```python
from build123d import *

# Parameters (mm, degrees)
SKETCH1_W           = 40
SKETCH1_H           = 45
BOSS_EXTRUDE1_DEPTH = 50
SHELL1_T            = -2.5
SKETCH3_W           = 40
SKETCH3_H           = 34.5
BOSS_EXTRUDE2_DEPTH = 10
SKETCH11_W          = 40
SKETCH11_H          = 5
CUT_EXTRUDE2_DEPTH  = 2.5
SKETCH12_W          = 37.5
SKETCH12_H          = 2
CUT_EXTRUDE3_DEPTH  = 1
SKETCH13_W          = 37.5
SKETCH13_H          = 2
CUT_EXTRUDE4_DEPTH  = 1
SKETCH15_R          = 1.5
CUT_EXTRUDE7_DEPTH  = 37
SKETCH16_R          = 1.5
CUT_EXTRUDE8_DEPTH  = 37
SKETCH17_R          = 3
CUT_EXTRUDE9_DEPTH  = 5
SKETCH19_W          = 15
SKETCH19_H          = 15
CUT_EXTRUDE10_DEPTH = 2.5


with BuildPart() as part:
    # Sketch1 → Boss-Extrude1 (new body)
    with BuildSketch(Plane(origin=(0, 0, 0), x_dir=(1, 0, 0), z_dir=(0, 1, 0))):
        with Locations((-14.888700463, -8.449653636)):
            Rectangle(SKETCH1_W, SKETCH1_H)
    extrude(amount=BOSS_EXTRUDE1_DEPTH)

    # Shell1
    shell1_openings = [part.faces().sort_by_distance(p)[0] for p in [
        (-14.888700463, 50, 8.449653636),
    ]]
    offset(amount=SHELL1_T, openings=shell1_openings, kind=Kind.INTERSECTION)

    # Sketch3 → Boss-Extrude2 (add)
    with BuildSketch(Plane(origin=(-32.388700463, 0, 0), x_dir=(0, 0, -1), z_dir=(1, 0, 0))):
        with Locations((-8.449653636, 19.75)):
            Rectangle(SKETCH3_W, SKETCH3_H)
    extrude(amount=BOSS_EXTRUDE2_DEPTH)

    # Sketch11 → Cut-Extrude2 (cut)
    with BuildSketch(Plane(origin=(-32.388700463, 0, 0), x_dir=(0, 0, -1), z_dir=(1, 0, 0))):
        with Locations((-8.449653636, 47.5)):
            Rectangle(SKETCH11_W, SKETCH11_H)
    extrude(amount=-CUT_EXTRUDE2_DEPTH, mode=Mode.SUBTRACT)

    # Sketch12 → Cut-Extrude3 (cut)
    with BuildSketch(Plane.XY.offset(-11.550346364)):
        with Locations((-16.138700463, 46)):
            Rectangle(SKETCH12_W, SKETCH12_H)
    extrude(amount=-CUT_EXTRUDE3_DEPTH, mode=Mode.SUBTRACT)

    # Sketch13 → Cut-Extrude4 (cut)
    with BuildSketch(Plane(origin=(0, 0, 28.449653636), x_dir=(-1, 0, 0), z_dir=(0, 0, -1))):
        with Locations((16.138700463, 46)):
            Rectangle(SKETCH13_W, SKETCH13_H)
    extrude(amount=-CUT_EXTRUDE4_DEPTH, mode=Mode.SUBTRACT)

    # Sketch15 → Cut-Extrude7 (cut)
    with BuildSketch(Plane(origin=(0, 37, 0), x_dir=(1, 0, 0), z_dir=(0, 1, 0))):
        with Locations(Location((-27.388700463, -15.949653636, 0), (0, 0, 270))):
            Circle(SKETCH15_R)
    extrude(amount=-CUT_EXTRUDE7_DEPTH, mode=Mode.SUBTRACT)

    # Sketch16 → Cut-Extrude8 (cut)
    with BuildSketch(Plane(origin=(0, 37, 0), x_dir=(1, 0, 0), z_dir=(0, 1, 0))):
        with Locations(Location((-27.388700463, -0.949653636, 0), (0, 0, 270))):
            Circle(SKETCH16_R)
    extrude(amount=-CUT_EXTRUDE8_DEPTH, mode=Mode.SUBTRACT)

    # Sketch17 → Cut-Extrude9 (cut)
    with BuildSketch(Plane.XZ):
        with Locations(Location((-27.388700463, 15.949653636, 0), (0, 0, 270))):
            Circle(SKETCH17_R)
        with Locations(Location((-27.388700463, 0.949653636, 0), (0, 0, 270))):
            Circle(SKETCH17_R)
    extrude(amount=-CUT_EXTRUDE9_DEPTH, mode=Mode.SUBTRACT)

    # Sketch19 → Cut-Extrude10 (cut)
    with BuildSketch(Plane.ZY.offset(-2.611299537)):
        with Locations((8.449653636, 10)):
            Rectangle(SKETCH19_W, SKETCH19_H)
    extrude(amount=-CUT_EXTRUDE10_DEPTH, mode=Mode.SUBTRACT)


solid = part.part
```
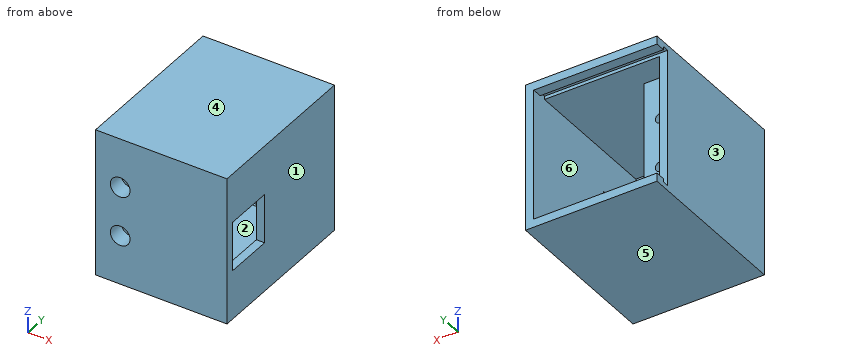
Work out the finished part from the listing and answer in its coordinate system (mm). Face numbers are marked on the shaded views. A direction names the side the tool comes from. Round coordinates to 2 decimals unless told otherwise and drop trailing zeros. Loops run counter-clockwise (first coordinate to the right, second up) from the corner with the lowest first, then second, coordinate; pieces in that order, holes last. Notation, with made-up numbers: (-23, -14.5) -> (24, -14.5) arc R29 cw to (24, 5.5) -> close; hole circle Ø7 at (-1, 87). An arc over 180 degrees is marked (long way). Write each question's results on one line, items separated by ' | '. Start each with the question number.
1. Section D-D (y = 9.5) is taken. Determine the outline of the cut face in (x, z), plus the area to 3 significant figures.
2. Section A-A (z = 10) is taken. Determine the outline of the cut face in (x, y).
3. Find the intervals of material crossed by probe 1 along X at (y, z) = (22, 16); probe 2 along Z at (x, y) = (-12.5, 11.5); probe 3 along X at (y, z) = (38, 0.5), in increasing order. Write a range as from..to.
4. Section C-C (y = 41) is taken. Determine the outline of the cut face in (x, z), plus the area to 3 significant figures.
5. Section B-B (x = -3) is taken. Determine the outline of the cut face in (y, z).
6. Given pin 1 Ø8 at (x, z) = (-2, 16.5) entering from +Y; pin 2 Ø3 at (x, z) = (-27.5, 11.5) entering from +Y; pin 3 Ø3 at (x, z) = (-28, 17) entering from -Y, each flat-ended and moving along its own axis, determine where each tip first touches the part or whether it passes through.
7. For a pull along Z with two mould halves and no side action, classify the marked faces 3, 4, 5 and 6 as +Z half, -Z half, draft (parallel to the pull), parting line (faces both ways), or undercut.
8. A tool of negligible diameter and unlimited length cuts with its end or side. For the marked faces 1 and 2, from which of +Z, -Z, +X, -X, +Y, -Y can it reach the whole face along a straight path? Write none if from no direction.
Evaluation:
1) outline: (-34.89, -14.05) -> (5.11, -14.05) -> (5.11, 0.95) -> (2.61, 0.95) -> (2.61, -11.55) -> (-22.39, -11.55) -> (-22.39, 28.45) -> (2.61, 28.45) -> (2.61, 15.95) -> (5.11, 15.95) -> (5.11, 30.95) -> (-34.89, 30.95) -> close; hole circle Ø3 at (-27.39, 0.95); hole circle Ø3 at (-27.39, 15.95) | area: 748 mm2
2) outline: (-34.89, 0) -> (5.11, 0) -> (5.11, 2.5) -> (-22.39, 2.5) -> (-22.39, 37) -> (-32.39, 37) -> (-32.39, 45) -> (-34.89, 45) -> close; (2.61, 17.5) -> (5.11, 17.5) -> (5.11, 50) -> (2.61, 50) -> close
3) probe 1: x = -34.89..-28.89, -25.89..-22.39, 2.61..5.11 | probe 2: z = -14.05..-11.55, 28.45..30.95 | probe 3: x = -34.89..-32.39, 2.61..5.11
4) outline: (-34.89, -14.05) -> (5.11, -14.05) -> (5.11, 30.95) -> (-34.89, 30.95) -> close; hole (-32.39, -11.55) -> (2.61, -11.55) -> (2.61, 28.45) -> (-32.39, 28.45) -> close | area: 400 mm2
5) outline: (0, -14.05) -> (50, -14.05) -> (50, -11.55) -> (47, -11.55) -> (47, -12.55) -> (45, -12.55) -> (45, -11.55) -> (2.5, -11.55) -> (2.5, 28.45) -> (45, 28.45) -> (45, 29.45) -> (47, 29.45) -> (47, 28.45) -> (50, 28.45) -> (50, 30.95) -> (0, 30.95) -> close
6) pin 1: stops at y = 2.5 | pin 2: stops at y = 37 | pin 3: stops at y = 5
7) face 3: draft | face 4: +Z half | face 5: -Z half | face 6: undercut
8) face 1: +Z, -Z, +X, +Y, -Y | face 2: +Y
